Input: part model. Units: mm. Frame: model coordinates. A direction names the side the tool comes from. Coordinates: 2 decimals unless noted, no trailing zeros. Order: outer loops, then holes, each group sorted by start corner. A loop starts at its lowest first (then second) coordinate and runs counter-clockwise, first axis right, second up. Notation, with made-up numbers: M 27,87 L 47,87 A22 ccw 47,118 Z; hole C 75.25,39 d10. An arc over 180 degrees is marked long. One line per item, written item: value.
```python
from build123d import *

# Parameters (mm, degrees)
F1_DEPTH     = 4.5
F3_DEPTH     = 2.75
F5_DEPTH     = 5
F6_T1_DEPTH  = 9.9607837082
F6_T3_DEPTH  = 12
F6_T6_ANGLE  = 90
F6_T8_ANGLE  = 90
F6_T10_ANGLE = 90
F6_T12_ANGLE = 90


# Not quite as in the source:
# - a fillet or chamfer that OpenCascade refuses, or shapes differently, is made with other operations: its cross-section is extruded or revolved along the edge and cut away or added


with BuildPart() as f1:
    # F0 (on Front) → F1 (new body, symmetric)
    with BuildSketch(Plane.XZ):
        with BuildLine():
            Line((6, 8), (-6, 8))
            ThreePointArc((-6, 8), (-8.1213203436, 7.1213203436), (-9, 5))
            Line((-9, 5), (-9, 0))
            Line((-9, 0), (9, 0))
            Line((9, 0), (9, 5))
            ThreePointArc((9, 5), (8.1213203436, 7.1213203436), (6, 8))
        make_face()
    extrude(amount=F1_DEPTH, both=True)

    # F2 (on Front) → F3 (cut, symmetric)
    with BuildSketch(Plane.XZ):
        Polygon((-24, 24), (-24, 0), (-6, 0), (-6, 6), (6, 6), (6, 0), (24, 0), (24, 24), align=None)
    extrude(amount=F3_DEPTH, both=True, mode=Mode.SUBTRACT)

    # F4 (on face) → F5 (cut)
    with BuildSketch(Plane(origin=(0, 0, 0), x_dir=(1, 0, 0), z_dir=(0, 0, -1))):
        with BuildLine():
            Line((4, -6), (4, 6))
            Line((4, 6), (1, 6))
            Line((1, 6), (1, 3.0521475958))
            Line((1, 3.0521475958), (-3.513030215, 1.4095389312))
            ThreePointArc((-3.513030215, 1.4095389312), (-4.4095389312, -0.513030215), (-2.486969785, -1.4095389312))
            Line((-2.486969785, -1.4095389312), (1, -0.1403857216))
            Line((1, -0.1403857216), (1, -6))
            Line((1, -6), (4, -6))
        make_face()
    extrude(amount=-F5_DEPTH, mode=Mode.SUBTRACT)

    # F6: fillet of radius 2 on 2 edges, made by hand

    # F6_s2 → F6_t1 (cut)
    with BuildSketch(Plane.XY.offset(-4.9607837082)):
        with BuildLine():
            ThreePointArc((9, 2.75), (8.3385621722, 4), (7.0156865167, 4.5))
            Line((7.0156865167, 4.5), (9, 4.5))
            Line((9, 4.5), (9, 2.75))
        make_face()
        with BuildLine():
            ThreePointArc((-7.0156865167, 4.5), (-8.3385621722, 4), (-9, 2.75))
            Line((-9, 2.75), (-9, 4.5))
            Line((-9, 4.5), (-7.0156865167, 4.5))
        make_face()
        with BuildLine():
            ThreePointArc((-7.0156865167, -4.5), (-8.3385621722, -4), (-9, -2.75))
            Line((-9, -2.75), (-9, -4.5))
            Line((-9, -4.5), (-7.0156865167, -4.5))
        make_face()
        with BuildLine():
            ThreePointArc((7.0156865167, -4.5), (8.3385621722, -4), (9, -2.75))
            Line((9, -2.75), (9, -4.5))
            Line((9, -4.5), (7.0156865167, -4.5))
        make_face()
    extrude(amount=F6_T1_DEPTH, mode=Mode.SUBTRACT)

    # F6_s4 → F6_t3 (cut)
    with BuildSketch(Plane.YZ.offset(-6)):
        with BuildLine():
            ThreePointArc((2.75, 8), (4, 7.3385621722), (4.5, 6.0156865167))
            Line((4.5, 6.0156865167), (4.5, 8))
            Line((4.5, 8), (2.75, 8))
        make_face()
        with BuildLine():
            ThreePointArc((-4.5, 6.0156865167), (-4, 7.3385621722), (-2.75, 8))
            Line((-2.75, 8), (-4.5, 8))
            Line((-4.5, 8), (-4.5, 6.0156865167))
        make_face()
    extrude(amount=F6_T3_DEPTH, mode=Mode.SUBTRACT)

    # F6_s5 → F6_t6 (revolve, cut)
    with BuildSketch(Plane.YZ.offset(-6)):
        with BuildLine():
            ThreePointArc((-4.5, 6.0156865167), (-4, 7.3385621722), (-2.75, 8))
            Line((-2.75, 8), (-4.5, 8))
            Line((-4.5, 8), (-4.5, 6.0156865167))
        make_face()
    revolve(axis=Axis((-6, -4.5, 5), (0, -1, 0)), revolution_arc=F6_T6_ANGLE, mode=Mode.SUBTRACT)

    # F6_s7 → F6_t8 (revolve, cut)
    with BuildSketch(Plane.XY.offset(5)):
        with BuildLine():
            ThreePointArc((9, 2.75), (8.3385621722, 4), (7.0156865167, 4.5))
            Line((7.0156865167, 4.5), (9, 4.5))
            Line((9, 4.5), (9, 2.75))
        make_face()
    revolve(axis=Axis((6, 4.5, 5), (0, -1, 0)), revolution_arc=F6_T8_ANGLE, mode=Mode.SUBTRACT)

    # F6_s9 → F6_t10 (revolve, cut)
    with BuildSketch(Plane.YZ.offset(-6)):
        with BuildLine():
            ThreePointArc((4.5, 6.0156865167), (4, 7.3385621722), (2.75, 8))
            Line((2.75, 8), (4.5, 8))
            Line((4.5, 8), (4.5, 6.0156865167))
        make_face()
    revolve(axis=Axis((-6, 4.5, 5), (0, -1, 0)), revolution_arc=F6_T10_ANGLE, mode=Mode.SUBTRACT)

    # F6_s11 → F6_t12 (revolve, cut)
    with BuildSketch(Plane.XY.offset(5)):
        with BuildLine():
            ThreePointArc((7.0156865167, -4.5), (8.3385621722, -4), (9, -2.75))
            Line((9, -2.75), (9, -4.5))
            Line((9, -4.5), (7.0156865167, -4.5))
        make_face()
    revolve(axis=Axis((6, -4.5, 5), (0, -1, 0)), revolution_arc=F6_T12_ANGLE, mode=Mode.SUBTRACT)


solid = f1.part
```
(1) Access query for faces 4 (the flat face through (0, 0, 6)), 5 (the flat face through (-0.768, 0.784, 2.465)), 6 (the flat face through (1, 2, 2)). Directions: +Z, -Z, +X, -X, +Y, -Y. A direction counts if a zero-diameter tool reaches every point of the face in a straight line with its end or side. Return the directions, or none.
Data:
face 4: +Z, +X, -X
face 5: -Z
face 6: -Z, +Y, -Y
(2) Cut plane A-A on z = 2.25. Output: boundary loops of the cut face in (x, y).
Data:
outline: M -9,-2.75 A2 ccw -7.02,-4.5 L 1,-4.5 L 1,-3.05 L -3.51,-1.41 A1.5 cw -2.49,1.41 L 1,0.14 L 1,4.5 L -7.02,4.5 A2 ccw -9,2.75 L -6,2.75 L -6,-2.75 Z; M 4,-4.5 L 7.02,-4.5 A2 ccw 9,-2.75 L 6,-2.75 L 6,2.75 L 9,2.75 A2 ccw 7.02,4.5 L 4,4.5 Z
(3) Ray query, line 1 (Y direction, x = -3.5, z = 3); line 2 (Y direction, x = -0.5, z = 3); line 3 (Z direction, x = 0, y = 2). Return the intervals inside material, ascending. Write a range as from..to.
Data:
line 1: y = -4.5..-1.41, 1.41..4.5
line 2: y = -4.5..-2.51, 0.69..4.5
line 3: z = 0..6
(4) Cut plane D-D on y = 1. Output: boundary loops of the cut face in (x, z).
Data:
outline: M -6,0 L -4.12,0 L -4.12,5 L -1.36,5 L -1.36,0 L 1,0 L 1,5 L 4,5 L 4,0 L 6,0 L 6,6 L -6,6 Z
(5) Draft query along Y for faces 1 (the cylindrical face through (-4.42, 0.48, 2.46)), 2 (the flat face through (0, -4.5, 3)), 3 (the flat face through (5, 0, 0)). Return one class per face: released by +Y, released by -Y, zero draft, split by the parting line, or undercut.
Data:
face 1: undercut
face 2: released by -Y
face 3: zero draft
(6) First-contact query: pin 1 (1 mm diameter, centred on y = 2, z = 5, fed in from +X); pin 2 (3 mm diameter, centred on y = 1, z = 2.5, fed in from -X); pin 3 (1.6 mm diameter, centred on x = 1.5, y = -0.5, fed in from +Z). Flat tips, straight axial feed; report the tip coordinate or a pass-through.
Data:
pin 1: stops at x = 6
pin 2: stops at x = -6
pin 3: stops at z = 6
(7) Cut plane B-B on x = -2. Output: boundary loops of the cut face in (y, z).
Data:
outline: M -4.5,0 L -1.96,0 L -1.96,5 L 1.23,5 L 1.23,0 L 4.5,0 L 4.5,6.02 A2 ccw 2.75,8 L 2.75,6 L -2.75,6 L -2.75,8 A2 ccw -4.5,6.02 Z
(8) Cut plane C-C on y = -0.75. Output: boundary loops of the cut face in (x, z), plus the area to 3 significant figures.
Data:
outline: M -6,0 L -4.3,0 L -4.3,5 L 4,5 L 4,0 L 6,0 L 6,6 L -6,6 Z
area: 30.5 mm2
